```python
from build123d import *

# Parameters (mm, degrees)
SKETCH1_R           = 1
BOSS_EXTRUDE1_DEPTH = 1
CHAMFER1_SIZE       = 0.2
CHAMFER2_SIZE       = 0.1


with BuildPart() as part:
    # Sketch1 → Boss-Extrude1 (new, symmetric)
    with BuildSketch(Plane.XY):
        with BuildLine():
            Line((-2, -17.5), (-2, 17.5))
            ThreePointArc((-2, 17.5), (0, 19.5), (2, 17.5))
            Line((2, 17.5), (2, -17.5))
            ThreePointArc((2, -17.5), (0, -19.5), (-2, -17.5))
        make_face()
        with Locations((0, 17.5)):
            Circle(SKETCH1_R, mode=Mode.SUBTRACT)
        with Locations((0, -17.5)):
            Circle(SKETCH1_R, mode=Mode.SUBTRACT)
    extrude(amount=BOSS_EXTRUDE1_DEPTH, both=True)

    # Chamfer1
    chamfer1_edges = [part.edges().sort_by_distance(p)[0] for p in [
        (0, 19.5, 1),
        (-2, 0, 1),
        (0, -19.5, 1),
        (-2, 0, -1),
        (0, 19.5, -1),
        (2, 0, -1),
        (0, -19.5, -1),
        (2, 0, 1),
    ]]
    chamfer(chamfer1_edges, length=CHAMFER1_SIZE)

    # Chamfer2
    chamfer2_edges = [part.edges().sort_by_distance(p)[0] for p in [
        (-1, 17.5, -1),
        (-1, 17.5, 1),
        (-1, -17.5, -1),
        (-1, -17.5, 1),
    ]]
    chamfer(chamfer2_edges, length=CHAMFER2_SIZE)


solid = part.part
```
For this review, take the finished solid that the model builds, in its own axes (mm). Round coordinates to 2 decimals unless told otherwise and drop trailing zeros. Loops run counter-clockwise (first coordinate to the right, second up) from the corner with the lowest first, then second, coordinate; pieces in that order, holes last.
Q1. To check wall thickness, follow line 1 along Y through (x, z) = (0, -0.45); line 2 along Y through (x, z) = (0.75, -0.5); line 3 along Y through (x, z) = (-1.15, 0.25). State the ranges of each line that lie inside material, in increasing order.
Result sheet:
line 1: y = -19.5 to -18.5, -16.5 to 16.5, 18.5 to 19.5
line 2: y = -19.35 to -18.16, -16.84 to 16.84, 18.16 to 19.35
line 3: y = -19.14 to 19.14
Q2. Add section A-A on x = 0. Write out the cut boundary in (y, z).
Result sheet:
outline: (-19.5, -0.8) - (-19.3, -1) - (-18.6, -1) - (-18.5, -0.9) - (-18.5, 0.9) - (-18.6, 1) - (-19.3, 1) - (-19.5, 0.8) - close; (-16.5, -0.9) - (-16.4, -1) - (16.4, -1) - (16.5, -0.9) - (16.5, 0.9) - (16.4, 1) - (-16.4, 1) - (-16.5, 0.9) - close; (18.5, -0.9) - (18.6, -1) - (19.3, -1) - (19.5, -0.8) - (19.5, 0.8) - (19.3, 1) - (18.6, 1) - (18.5, 0.9) - close
Q3. Add section B-B on z = 0.2. Write out the cut boundary in (x, y).
Result sheet:
outline: (-2, -17.5) arc R2 ccw to (2, -17.5) - (2, 17.5) arc R2 ccw to (-2, 17.5) - close; hole circle Ø2 at (0, -17.5); hole circle Ø2 at (0, 17.5)
Q4. Mouldability with a two-part tool opening along X and no side actions: class faces 1 (the face through (0, 0, -1)), 2 (the face through (0, 19.5, 0)), 3 (the face through (-0.217, -18.476, -0.013)), 4 (the face through (-2, 0, 0)) as +X half, -X half, draft (parallel to the pull), parting line (faces both ways), or undercut.
Result sheet:
face 1: draft
face 2: parting line
face 3: undercut
face 4: -X half
